Geometry: final body of the model. Coordinates: model frame, mm. Face numbers are marked on the shaded views. Give positions to 0.01 mm unless a question says otherwise; leave off trailing zeros. Loops run counter-clockwise (first coordinate to the right, second up) from the corner with the lowest first, then second, coordinate; pieces in that order, holes last.
1. Draft query along Z for the marked faces 1, 2 and 3. Return one class per face: +Z half, -Z half, draft (parallel to the pull), parting line (faces both ways), or undercut.
2. Material intervals for line 1 along Z through (x, y) = (-0.25, 0.7); line 2 along Z through (x, y) = (-0.5, 0.2); line 3 along Z through (x, y) = (2.5, 1.4), sorted ascending.
3. First-contact query: P1, Ø1.2, axis at y = 0.5, z = 6, coming from the -X side (3 decimals); P2, Ø0.9, axis at x = 0, z = 4.5, coming from the +Y side; P3, Ø0.5, axis at y = 0.5, z = 5, coming from the +X side (3 decimals); P4, Ø1, axis at y = 2, z = -2.5, coming from the -X side (3 decimals). Flat tips, straight axial feed; report the tip coordinate or a pass-through.
4. Section D-D, the plane x = -2. Output: boundary loops of the cut face in (y, z), then the cut area to 3 significant figures.
5. Section C-C, the plane y = 0.65. Output: boundary loops of the cut face in (x, z) (3 decimals), then the cut area to 3 significant figures.
6. Section B-B, the plane x = 0. Output: boundary loops of the cut face in (y, z), then the cut area to 3 significant figures.
7. Section A-A, the plane z = 4.75. Output: boundary loops of the cut face in (x, y) (3 decimals).
from build123d import *

# Parameters (mm, degrees)
SKETCH1_W           = 6.35
SKETCH1_H           = 8
BOSS_EXTRUDE1_DEPTH = 2
FILLET1_R           = 0.15
BOSS_EXTRUDE2_DEPTH = 0.425
BOSS_EXTRUDE3_START = -0.5
BOSS_EXTRUDE3_DEPTH = 0.85


with BuildPart() as part:
    # Sketch1 → Boss-Extrude1 (new body)
    with BuildSketch(Plane(origin=(0, 0, 0), x_dir=(1, 0, 0), z_dir=(0, 1, 0))):
        Rectangle(SKETCH1_W, SKETCH1_H)
    extrude(amount=BOSS_EXTRUDE1_DEPTH)

    # Fillet1
    fillet1_edges = [part.edges().sort_by_distance(p)[0] for p in [
        (3.175, 2, 0),
        (0, 2, -4),
        (-3.175, 2, 0),
        (0, 2, 4),
        (-3.175, 1, -4),
        (3.175, 1, -4),
        (3.175, 1, 4),
        (-3.175, 1, 4),
    ]]
    fillet(fillet1_edges, radius=FILLET1_R)

    # Sketch2 → Boss-Extrude2 (add, symmetric)
    with BuildSketch(Plane(origin=(0, 0, 0), x_dir=(0, 0, -1), z_dir=(1, 0, 0))):
        with BuildLine():
            Line((-4, 1.5), (-5.1, 1.5))
            ThreePointArc((-5.1, 1.5), (-5.382842712, 1.382842712), (-5.5, 1.1))
            Line((-5.5, 1.1), (-5.5, 0.4))
            ThreePointArc((-5.5, 0.4), (-5.382842712, 0.117157288), (-5.1, 0))
            Line((-5.1, 0), (-4.4, 0))
            Line((-4.4, 0), (-4.4, 0.4))
            Line((-4.4, 0.4), (-5.1, 0.4))
            Line((-5.1, 0.4), (-5.1, 1.1))
            Line((-5.1, 1.1), (-4, 1.1))
            Line((-4, 1.1), (-4, 1.5))
        make_face()
    extrude(amount=BOSS_EXTRUDE2_DEPTH, both=True)

    # Sketch3 → Boss-Extrude3 (add)
    with BuildSketch(Plane(origin=(3.175, 0, 0), x_dir=(0, 0, -1), z_dir=(1, 0, 0)).offset(BOSS_EXTRUDE3_START)):
        with BuildLine():
            Line((-4, 1.5), (-5.473547717, 1.5))
            ThreePointArc((-5.473547717, 1.5), (-5.703670661, 1.427174923), (-5.85, 1.235217152))
            Line((-5.85, 1.235217152), (-6.15, 0.4))
            Line((-6.15, 0.4), (-7, 0.4))
            Line((-7, 0.4), (-7, 0))
            Line((-7, 0), (-6.15, 0))
            ThreePointArc((-6.15, 0), (-5.919877056, 0.072825077), (-5.773547717, 0.264782848))
            Line((-5.773547717, 0.264782848), (-5.473547717, 1.1))
            Line((-5.473547717, 1.1), (-4, 1.1))
            Line((-4, 1.1), (-4, 1.5))
        make_face()
    boss_extrude3 = extrude(amount=-BOSS_EXTRUDE3_DEPTH)

    # Mirror1: Boss-Extrude3 across plane
    add(boss_extrude3.mirror(Plane(origin=(0, 0, 0), x_dir=(0, 0, 1), z_dir=(1, 0, 0))))


solid = part.part
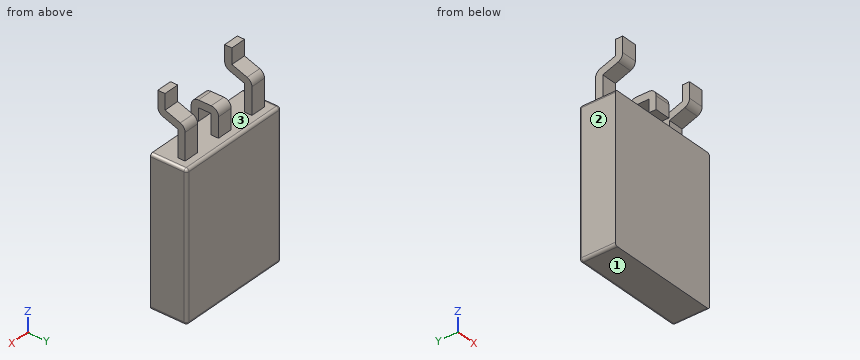
Answers below:
1. face 1: -Z half
1. face 2: draft
1. face 3: undercut
2. line 1: z = -4 to 4, 5.1 to 5.5
2. line 2: z = -4 to 4
2. line 3: z = -4 to 5.74
3. P1: stops at x = -2.675
3. P2: stops at y = 1.5
3. P3: stops at x = 0.425
3. P4: stops at x = -3.175
4. outline: (0, -4) - (1.85, -4) arc R0.15 ccw to (2, -3.85) - (2, 3.85) arc R0.15 ccw to (1.85, 4) - (1.5, 4) - (1.5, 5.47) arc R0.4 ccw to (1.24, 5.85) - (0.4, 6.15) - (0.4, 7) - (0, 7) - (0, 6.15) arc R0.4 ccw to (0.26, 5.77) - (1.1, 5.47) - (1.1, 4) - (0, 4) - close
4. area: 17.5 mm2
5. outline: (-3.175, -3.85) arc R0.15 ccw to (-3.025, -4) - (3.025, -4) arc R0.15 ccw to (3.175, -3.85) - (3.175, 3.85) arc R0.15 ccw to (3.025, 4) - (-3.025, 4) arc R0.15 ccw to (-3.175, 3.85) - close; (-2.675, 5.635) - (-1.825, 5.635) - (-1.825, 6.06) - (-2.675, 6.06) - close; (-0.425, 5.1) - (0.425, 5.1) - (0.425, 5.5) - (-0.425, 5.5) - close; (1.825, 5.635) - (2.675, 5.635) - (2.675, 6.06) - (1.825, 6.06) - close
5. area: 51.8 mm2
6. outline: (0, -4) - (1.85, -4) arc R0.15 ccw to (2, -3.85) - (2, 3.85) arc R0.15 ccw to (1.85, 4) - (1.5, 4) - (1.5, 5.1) arc R0.4 ccw to (1.1, 5.5) - (0.4, 5.5) arc R0.4 ccw to (0, 5.1) - (0, 4.4) - (0.4, 4.4) - (0.4, 5.1) - (1.1, 5.1) - (1.1, 4) - (0, 4) - close
6. area: 17.2 mm2
7. outline: (-2.675, 1.1) - (-1.825, 1.1) - (-1.825, 1.5) - (-2.675, 1.5) - close; (-0.425, 0) - (0.425, 0) - (0.425, 0.4) - (-0.425, 0.4) - close; (-0.425, 1.1) - (0.425, 1.1) - (0.425, 1.5) - (-0.425, 1.5) - close; (1.825, 1.1) - (2.675, 1.1) - (2.675, 1.5) - (1.825, 1.5) - close
